Work out the finished part from the listing and answer in its coordinate system (mm). A direction names the side the tool comes from. Round coordinates to 2 decimals unless told otherwise and drop trailing zeros. Loops run counter-clockwise (first coordinate to the right, second up) from the corner with the lowest first, then second, coordinate; pieces in that order, holes last.
```python
from build123d import *

# Parameters (mm, degrees)
IZIM1_W                     = 121.550964813
IZIM1_H                     = 79.400227015
IZIM1_W_2                   = 108.562656073
IZIM1_H_2                   = 67.392167991
Y_KSEKLIK_EKSTR_ZYON1_DEPTH = 68.58
IZIM2_W                     = 108.665778405
IZIM2_H                     = 2.839609685
Y_KSEKLIK_EKSTR_ZYON3_DEPTH = 67.31
IZIM4_W                     = 43.769026383
IZIM4_H                     = 34.779664875
KES_EKSTR_ZYON3_DEPTH       = 51.308
RADYUS1_R                   = 10
RADYUS2_R                   = 10
KES_EKSTR_ZYON6_DEPTH       = 25.4
Y_KSEKLIK_EKSTR_ZYON4_DEPTH = 4.572


with BuildPart() as part:
    # Çizim1 → Yükseklik-Ekstrüzyon1 (new body)
    with BuildSketch(Plane.XY):
        with Locations((3.983010787, 3.063280364)):
            Rectangle(IZIM1_W, IZIM1_H)
        with Locations((3.860479571, 3.185811577)):
            Rectangle(IZIM1_W_2, IZIM1_H_2, mode=Mode.SUBTRACT)
    extrude(amount=Y_KSEKLIK_EKSTR_ZYON1_DEPTH)

    # Çizim2 → Yükseklik-Ekstrüzyon3 (add)
    with BuildSketch(Plane(origin=(0, -30.510272418, 0), x_dir=(1, 0, 0), z_dir=(0, 1, 0))):
        with Locations((3.70835341, -1.557090266)):
            Rectangle(IZIM2_W, IZIM2_H)
    extrude(amount=Y_KSEKLIK_EKSTR_ZYON3_DEPTH)

    # Çizim4 → Kes-Ekstrüzyon3 (cut)
    with BuildSketch(Plane(origin=(0, 0, 0.137285424), x_dir=(-1, 0, 0), z_dir=(0, 0, -1))):
        with Locations((-2.08713858, 8.765719608)):
            Rectangle(IZIM4_W, IZIM4_H)
    extrude(amount=-KES_EKSTR_ZYON3_DEPTH, mode=Mode.SUBTRACT)

    # Radyus1
    # the kernel refuses this fillet: 10 mm, written as the material it takes off along each edge
    with BuildSketch(Plane(origin=(64.758493193, -36.636833144, -25), x_dir=(0, 1, 0), z_dir=(0, 0, 1)), Plane(origin=(64.758493193, 42.763393871, -25), x_dir=(-1, 0, 0), z_dir=(0, 0, 1))) as radyus1_piece_1:
        with BuildLine():
            CenterArc((RADYUS1_R, RADYUS1_R), RADYUS1_R, 180, 90)
            Line((0, RADYUS1_R), (0, 0))
            Line((0, 0), (RADYUS1_R, 0))
        make_face()
    extrude(amount=118.58, mode=Mode.SUBTRACT)
    with BuildSketch(Plane(origin=(64.758493193, 67.763393871, 68.58), x_dir=(0, 0, -1), z_dir=(0, -1, 0))) as radyus1_piece_2:
        with BuildLine():
            CenterArc((RADYUS1_R, -RADYUS1_R), RADYUS1_R, 90, 90)
            Line((0, -RADYUS1_R), (0, 0))
            Line((0, 0), (RADYUS1_R, 0))
        make_face()
    extrude(amount=129.400227015, mode=Mode.SUBTRACT)
    with BuildSketch(Plane(origin=(64.758493193, 67.763393871, 0), x_dir=(0, 0, 1), z_dir=(0, -1, 0))) as radyus1_piece_3:
        with BuildLine():
            CenterArc((RADYUS1_R, RADYUS1_R), RADYUS1_R, 180, 90)
            Line((0, RADYUS1_R), (0, 0))
            Line((0, 0), (RADYUS1_R, 0))
        make_face()
    extrude(amount=129.400227015, mode=Mode.SUBTRACT)

    # Radyus2
    # the kernel refuses this fillet: 10 mm, written as the material it takes off along each edge
    with BuildSketch(Plane(origin=(-56.79247162, 42.763393871, -25), x_dir=(1, 0, 0), z_dir=(0, 0, 1)), Plane(origin=(-56.79247162, -36.636833144, -25), x_dir=(0, 1, 0), z_dir=(0, 0, 1))) as radyus2_piece_1:
        with BuildLine():
            CenterArc((RADYUS2_R, -RADYUS2_R), RADYUS2_R, 90, 90)
            Line((0, -RADYUS2_R), (0, 0))
            Line((0, 0), (RADYUS2_R, 0))
        make_face()
    extrude(amount=118.58, mode=Mode.SUBTRACT)
    with BuildSketch(Plane(origin=(-56.79247162, -61.636833144, 68.58), x_dir=(1, 0, 0), z_dir=(0, 1, 0))) as radyus2_piece_2:
        with BuildLine():
            CenterArc((RADYUS2_R, RADYUS2_R), RADYUS2_R, 180, 90)
            Line((0, RADYUS2_R), (0, 0))
            Line((0, 0), (RADYUS2_R, 0))
        make_face()
    extrude(amount=129.400227015, mode=Mode.SUBTRACT)
    with BuildSketch(Plane(origin=(-56.79247162, -61.636833144, 0), x_dir=(1, 0, 0), z_dir=(0, 1, 0))) as radyus2_piece_3:
        with BuildLine():
            CenterArc((RADYUS2_R, -RADYUS2_R), RADYUS2_R, 90, 90)
            Line((0, -RADYUS2_R), (0, 0))
            Line((0, 0), (RADYUS2_R, 0))
        make_face()
    extrude(amount=129.400227015, mode=Mode.SUBTRACT)

    # Çizim5 → Kes-Ekstrüzyon6 (cut)
    with BuildSketch(Plane(origin=(0, 42.763393871, 0), x_dir=(1, 0, 0), z_dir=(0, 1, 0))):
        with BuildLine():
            Line((-46.423230595, -35.751971692), (55.012749139, -35.751971692))
            ThreePointArc((55.012749139, -35.751971692), (56.029772925, -36.768995478), (55.012749139, -37.786019263))
            Line((55.012749139, -37.786019263), (-46.423230595, -37.786019263))
            ThreePointArc((-46.423230595, -37.786019263), (-47.44025438, -36.768995478), (-46.423230595, -35.751971692))
        make_face()
        with BuildLine():
            Line((-46.550358568, -42.998266165), (54.885621166, -42.998266165))
            ThreePointArc((54.885621166, -42.998266165), (55.902644952, -44.015289951), (54.885621166, -45.032313737))
            Line((54.885621166, -45.032313737), (-46.550358568, -45.032313737))
            ThreePointArc((-46.550358568, -45.032313737), (-47.567382354, -44.015289951), (-46.550358568, -42.998266165))
        make_face()
        with BuildLine():
            Line((-46.677486541, -39.438682915), (54.758493193, -39.438682915))
            ThreePointArc((54.758493193, -39.438682915), (55.775516978, -40.455706701), (54.758493193, -41.472730487))
            Line((54.758493193, -41.472730487), (-46.677486541, -41.472730487))
            ThreePointArc((-46.677486541, -41.472730487), (-47.694510327, -40.455706701), (-46.677486541, -39.438682915))
        make_face()
    extrude(amount=-KES_EKSTR_ZYON6_DEPTH, mode=Mode.SUBTRACT)

    # Çizim6 → Yükseklik-Ekstrüzyon4 (add)
    with BuildSketch(Plane(origin=(0, -36.636833144, 0), x_dir=(-1, 0, 0), z_dir=(0, -1, 0))):
        with BuildLine():
            Line((-46.87100271, -4.227005014), (-46.87100271, -64.014742354))
            ThreePointArc((-46.87100271, -64.014742354), (-49.504404567, -66.64814421), (-52.137806423, -64.014742354))
            Line((-52.137806423, -64.014742354), (-52.137806423, -4.227005014))
            ThreePointArc((-52.137806423, -4.227005014), (-49.504404567, -1.593603158), (-46.87100271, -4.227005014))
        make_face()
        with BuildLine():
            Line((44.301980946, -4.525434052), (44.301980946, -64.313171393))
            ThreePointArc((44.301980946, -64.313171393), (41.66857909, -66.946573249), (39.035177234, -64.313171393))
            Line((39.035177234, -64.313171393), (39.035177234, -4.525434052))
            ThreePointArc((39.035177234, -4.525434052), (41.66857909, -1.892032196), (44.301980946, -4.525434052))
        make_face()
    extrude(amount=Y_KSEKLIK_EKSTR_ZYON4_DEPTH)


solid = part.part
```
1. Consider probe 1 along Z at (x, y) = (-19, 38); probe 2 along X at (y, z) = (11, 52); probe 3 along Y at (x, z) = (-12.5, 29). Determine where each line is inside the solid, lowest interval first.
Answer key:
probe 1: z = 0 to 35.75, 37.79 to 39.44, 41.47 to 43, 45.03 to 68.58
probe 2: x = -56.79 to -50.42, 58.14 to 64.76
probe 3: y = -36.64 to -30.51, 36.88 to 42.76
2. Determine the mould class of faces 4 (the face through (-53.94, -33.63, 33.81)), 5 (the face through (-41.726, -38.891, 66.946)), 6 (the face through (3, 36.882, 34)) for opening direction Y: +Y half, -Y half, draft (parallel to the pull), parting line (faces both ways), or undercut.
Answer key:
face 4: -Y half
face 5: draft
face 6: undercut
3. Find section A-A (x = -26.5). Write down the section's boundary in (y, z), then the cut area to 3 significant figures.
Answer key:
outline: (-36.64, 0) - (-30.51, 0) - (-30.51, 0.14) - (36.8, 0.14) - (36.8, 2.98) - (-30.51, 2.98) - (-30.51, 68.58) - (-36.64, 68.58) - close; (36.88, 0) - (42.76, 0) - (42.76, 35.75) - (36.88, 35.75) - close; (36.88, 37.79) - (42.76, 37.79) - (42.76, 39.44) - (36.88, 39.44) - close; (36.88, 41.47) - (42.76, 41.47) - (42.76, 43) - (36.88, 43) - close; (36.88, 45.03) - (42.76, 45.03) - (42.76, 68.58) - (36.88, 68.58) - close
area: 979 mm2
4. Which of the six approach directions +Z, -Z, +X, -X, +Y, -Y give full straight-line access (tool end or side, diameter ignored) to faces 1 (the face through (58.142, 3, 34)), 2 (the face through (49.562, -38.891, 1.594)), 3 (the face through (5, 40, 45.032))?
Answer key:
face 1: +Z, -Z
face 2: -Z, -Y
face 3: +Y
5. Find section D-D (x = 3). Write down the section's boundary in (y, z).
Answer key:
outline: (-36.64, 0) - (-30.51, 0) - (-30.51, 0.14) - (-8.62, 0.14) - (-8.62, 2.98) - (-30.51, 2.98) - (-30.51, 68.58) - (-36.64, 68.58) - close; (26.16, 0.14) - (36.8, 0.14) - (36.8, 2.98) - (26.16, 2.98) - close; (36.88, 0) - (42.76, 0) - (42.76, 35.75) - (36.88, 35.75) - close; (36.88, 37.79) - (42.76, 37.79) - (42.76, 39.44) - (36.88, 39.44) - close; (36.88, 41.47) - (42.76, 41.47) - (42.76, 43) - (36.88, 43) - close; (36.88, 45.03) - (42.76, 45.03) - (42.76, 68.58) - (36.88, 68.58) - close
6. Find section C-C (z = 49). Write down the section's boundary in (x, y), then the cut area to 3 significant figures.
Answer key:
outline: (-56.79, -26.64) arc R10 ccw to (-46.79, -36.64) - (-44.3, -36.64) - (-44.3, -41.21) - (-39.04, -41.21) - (-39.04, -36.64) - (46.87, -36.64) - (46.87, -41.21) - (52.14, -41.21) - (52.14, -36.64) - (54.76, -36.64) arc R10 ccw to (64.76, -26.64) - (64.76, 32.76) arc R10 ccw to (54.76, 42.76) - (-46.79, 42.76) arc R10 ccw to (-56.79, 32.76) - close; hole (-50.42, -30.51) - (58.14, -30.51) - (58.14, 36.88) - (-50.42, 36.88) - close
area: 2,300 mm2
7. Find section B-B (y = 19). Write down the section's boundary in (x, z), then the cut area to 3 significant figures.
Answer key:
outline: (-56.79, 10) arc R10 ccw to (-48.44, 0.14) - (-19.8, 0.14) - (-19.8, 2.98) - (-50.42, 2.98) - (-50.42, 67.9) arc R10 ccw to (-56.79, 58.58) - close; (23.97, 0.14) - (56.41, 0.14) arc R10 ccw to (58.04, 0.55) - (58.04, 2.98) - (23.97, 2.98) - close; (58.14, 0.59) arc R10 ccw to (64.76, 10) - (64.76, 58.58) arc R10 ccw to (58.14, 67.99) - close
area: 991 mm2
8. Given pin 1 (5 mm diameter, centred on y = -38, z = 37.5, fed in from -X); pin 2 (3 mm diameter, centred on x = 10, z = 1.5, fed in from -Y); pin 3 (1.9 mm diameter, centred on y = -5, z = 1.5, fed in from +X); pin 4 (2 mm diameter, centred on x = -9.5, y = 24.5, fed in from +Z), each flat-ended and moving along its own axis, determine where each tip first touches the part or whether it passes through.
Answer key:
pin 1: stops at x = -51.42
pin 2: stops at y = -36.64
pin 3: stops at x = 61.32
pin 4: passes through
